Input: dimensioned drawing with shaded views. Units: mm. Origin: part minimum x, y, z. A direction names the side the tool comes from. Coordinates: 2 decimals unless noted, no trailing zeros. Order: outer loops, then holes, each group sorted by start corner. A loop starts at its lowest first (then second) coordinate and runs counter-clockwise, first axis right, second up. Notation, with made-up numbers: (43.5, 2.25) -> (86.5, 2.25) arc R21 ccw to (86.5, 40.25) -> close; hole circle Ø2 at (-9, 71). An arc over 180 degrees is marked (long way). Answer in a Markdown table with one row per item. Add a question column.
1) Contact query for flat-ended pins moving along their axis: P1, Ø8, axis at x = 12, z = 6.5, coming from the +Y side; P2, Ø8, axis at y = 9.5, z = 7.5, coming from the -X side; P3, Ø5, axis at y = 16.5, z = 8.5, coming from the -X side. Output: stop coordinate, or through.
2) Ray query, line 1 (Z direction, x = 36.5, y = 45); line 2 (Z direction, x = 33.5, y = 8.5); line 3 (X direction, y = 14.5, z = 9). Return the intervals inside material, ascending. Write a range as from..to.
3) Section query C-C on z = 10.25. Return the cut outline in (x, y), then the cut area to 3 significant figures.
4) Set-up query: the marked faces 1, 2 and 3. Return all of +Z, -Z, +X, -X, +Y, -Y with unobstructed straight access to the full face (end or side cutting, diameter ignored); none if empty.
5) Section query A-A on y = 25. Return the cut outline in (x, z).
6) Section query D-D on x = 44.5. Return the cut outline in (y, z).
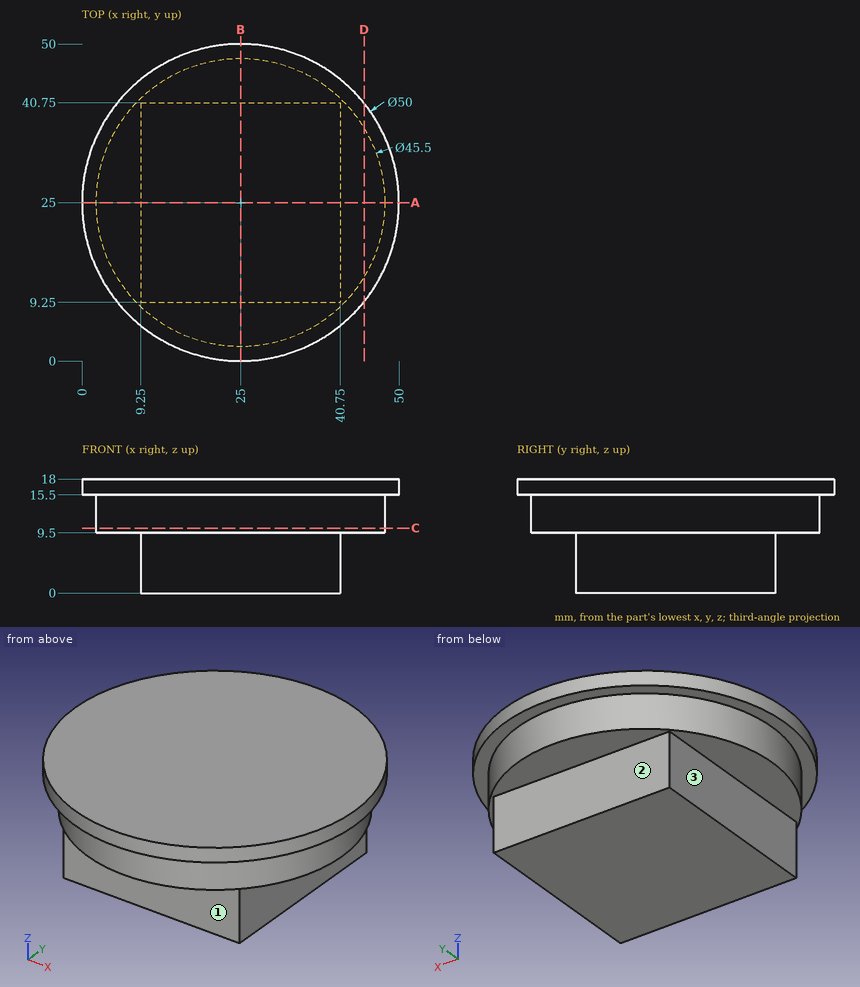
Result:
| question | item | result |
|---|---|---|
| 1 | P1 | y = 45.26 |
| 1 | P2 | x = 5.69 |
| 1 | P3 | x = 3.11 |
| 2 | line 1 | 15.5..18 |
| 2 | line 2 | 9.5..18 |
| 2 | line 3 | 9.25..40.75 |
| 3 | outline | circle Ø45.5 at (25, 25) |
| 3 | area | 1,630 mm2 |
| 4 | face 1 | -Z, +X, -X, -Y |
| 4 | face 2 | -Z, +X, -X, +Y |
| 4 | face 3 | -Z, -X, +Y, -Y |
| 5 | outline | (0, 15.5) -> (2.25, 15.5) -> (2.25, 9.5) -> (9.25, 9.5) -> (9.25, 0) -> (40.75, 0) -> (40.75, 9.5) -> (47.75, 9.5) -> (47.75, 15.5) -> (50, 15.5) -> (50, 18) -> (0, 18) -> close |
| 6 | outline | (9.36, 15.5) -> (13.28, 15.5) -> (13.28, 9.5) -> (36.72, 9.5) -> (36.72, 15.5) -> (40.64, 15.5) -> (40.64, 18) -> (9.36, 18) -> close |
